from build123d import *

# Parameters (mm, degrees)
SKETCH_1_R      = 3.3
SKETCH_1_R_2    = 37.8
EXTRUDE_1_DEPTH = 3


with BuildPart() as part:
    # 草图1 → 凸台-拉伸1 (new body)
    with BuildSketch(Plane.XY):
        with BuildLine():
            Line((0, -47), (235, -47))
            ThreePointArc((235, -47), (282, 0), (235, 47))
            Line((235, 47), (0, 47))
            ThreePointArc((0, 47), (-47, 0), (0, -47))
        make_face()
        with Locations((16.264045876, -39.264880132)):
            Circle(SKETCH_1_R, mode=Mode.SUBTRACT)
        with Locations((39.264880132, -16.264045876)):
            Circle(SKETCH_1_R, mode=Mode.SUBTRACT)
        with Locations((39.264880132, 16.264045876)):
            Circle(SKETCH_1_R, mode=Mode.SUBTRACT)
        with Locations((16.264045876, 39.264880132)):
            Circle(SKETCH_1_R, mode=Mode.SUBTRACT)
        with Locations((-16.264045876, 39.264880132)):
            Circle(SKETCH_1_R, mode=Mode.SUBTRACT)
        with Locations((-39.264880132, 16.264045876)):
            Circle(SKETCH_1_R, mode=Mode.SUBTRACT)
        with Locations((-39.264880132, -16.264045876)):
            Circle(SKETCH_1_R, mode=Mode.SUBTRACT)
        with Locations((-16.264045876, -39.264880132)):
            Circle(SKETCH_1_R, mode=Mode.SUBTRACT)
        with Locations((251.264045876, -39.264880132)):
            Circle(SKETCH_1_R, mode=Mode.SUBTRACT)
        with Locations((274.264880132, -16.264045876)):
            Circle(SKETCH_1_R, mode=Mode.SUBTRACT)
        with Locations((274.264880132, 16.264045876)):
            Circle(SKETCH_1_R, mode=Mode.SUBTRACT)
        with Locations((251.264045876, 39.264880132)):
            Circle(SKETCH_1_R, mode=Mode.SUBTRACT)
        with Locations((218.735954124, 39.264880132)):
            Circle(SKETCH_1_R, mode=Mode.SUBTRACT)
        with Locations((195.735119868, 16.264045876)):
            Circle(SKETCH_1_R, mode=Mode.SUBTRACT)
        with Locations((195.735119868, -16.264045876)):
            Circle(SKETCH_1_R, mode=Mode.SUBTRACT)
        with Locations((218.735954124, -39.264880132)):
            Circle(SKETCH_1_R, mode=Mode.SUBTRACT)
        Circle(SKETCH_1_R_2, mode=Mode.SUBTRACT)
        with Locations((235, 0)):
            Circle(SKETCH_1_R_2, mode=Mode.SUBTRACT)
    extrude(amount=EXTRUDE_1_DEPTH)


solid = part.part
Can you work these out from the model? Positions are in its coordinate system, mm. Coordinates: 2 decimals unless noted, no trailing zeros. Write each loop counter-clockwise with the first axis right and the second up, starting at its lowest first coordinate (ties: lowest second). Pieces come first, ordered by that corner, then holes. Notation, with made-up numbers: (37.5, 80.5) - (42.5, 80.5) arc R29 cw to (42.5, 102.5) - close; hole circle Ø11 at (10.5, -22.75). An arc over 180 degrees is marked (long way). Return JSON: item names as keys, results as strings. Group by question number.
Item 1: If we section it at B-B (x = 207.5): Write out the boundary of the cut face in (y, z).
Item 2: We'd pull the mould along Y, two halves only. Please class faces 1 (the face through (281.99, -1.03, 1.48)), 2 (the face through (36.054, 11.354, 1.479)), 3 (the face through (115, 1, 3)): pulls with the +Y half, pulls with the -Y half, needs draft (parallel to the pull), parting line crosses it, or undercut.
Item 3: If we section it at D-D (y = 29): Write out the boundary of the cut face in (x, z), then the cut area to 3 significant figures.
Item 4: I'm going to push flat-ended pins straight in: pin 1 Ø1.5 at (y, z) = (-20.5, 1) entering from -X; pin 2 Ø1.5 at (y, z) = (-23.5, 1) entering from +X; pin 3 Ø1 at (y, z) = (21, 1) entering from +X; pin 4 Ø5.5 at (x, y) = (218.74, -39.26) entering from -Z. Where does each tip first touch, or does it pass through?
Item 5: If we section it at A-A (y = 0): Write out the boundary of the cut face in (x, z).
Item 6: If we section it at C-C (z = 0.85): Count the separate pieces of the cut face and the enclosed holes in it, then the cut area to 3 significant figures.
Item 7: Please list where these lines run through material, in increasing order: probe 1 along X at (y, z) = (11, 2.45); probe 2 along Y at (x, z) = (0, 0.8); probe 3 along X at (y, z) = (24, 1.95).
Return value:
{
 "1": {"outline": "(-47, 0) - (-25.93, 0) - (-25.93, 3) - (-47, 3) - close; (25.93, 0) - (47, 0) - (47, 3) - (25.93, 3) - close"},
 "2": {"face 1": "parting line crosses it", "face 2": "undercut", "face 3": "needs draft"},
 "3": {"outline": "(-36.99, 0) - (-24.25, 0) - (-24.25, 3) - (-36.99, 3) - close; (24.25, 0) - (210.75, 0) - (210.75, 3) - (24.25, 3) - close; (259.25, 0) - (271.99, 0) - (271.99, 3) - (259.25, 3) - close", "area": "636 mm^2"},
 "4": {"pin 1": "stops at x = -42.65", "pin 2": "stops at x = 276.13", "pin 3": "stops at x = 277.29", "pin 4": "passes through"},
 "5": {"outline": "(-47, 0) - (-37.8, 0) - (-37.8, 3) - (-47, 3) - close; (37.8, 0) - (197.2, 0) - (197.2, 3) - (37.8, 3) - close; (272.8, 0) - (282, 0) - (282, 3) - (272.8, 3) - close"},
 "6": {"separate pieces": "1", "enclosed holes": "18", "area": "19,500 mm^2"},
 "7": {"probe 1": "x = -45.69 to -36.16, 36.16 to 198.84, 271.16 to 280.69", "probe 2": "y = -47 to -37.8, 37.8 to 47", "probe 3": "x = -40.41 to -29.2, 29.2 to 205.8, 264.2 to 275.41"}
}
